Geometry check sheet. Reference: the model listing, model coordinates, mm. Face numbers are marked on the shaded views. A direction names the side the tool comes from. Round coordinates to 2 decimals unless told otherwise and drop trailing zeros. Write each loop counter-clockwise with the first axis right and the second up, starting at its lowest first coordinate (ties: lowest second). Pieces come first, ordered by that corner, then holes. Notation, with made-up numbers: (11.25, 0) -> (41.25, 0) arc R12 ccw to (41.25, 5) -> close; hole circle Ø6 at (43, 31.25). An arc over 180 degrees is marked (long way). Use a Markdown table: item, result.
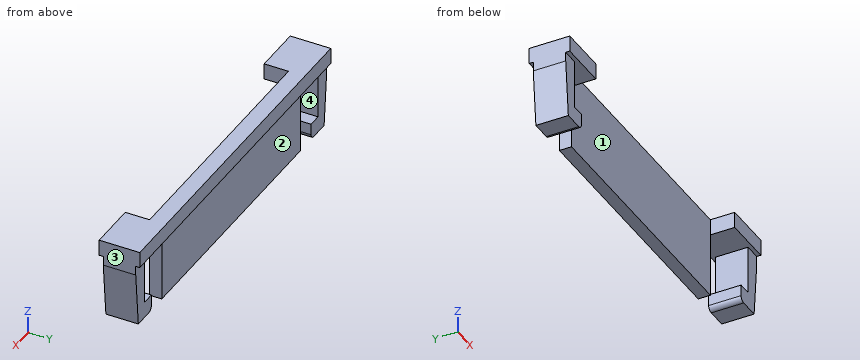
```python
from build123d import *

# Parameters (mm, degrees)
SKETCH1_W             = 22
SKETCH1_H             = 2.5
BOSS_EXTRUDE1_DEPTH   = 5
SKETCH2_W             = 22
SKETCH2_H             = 0.25
CUT_EXTRUDE1_DEPTH    = 4
SKETCH3_W             = 2
SKETCH3_H             = 2
CUT_EXTRUDE2_DEPTH    = 4
SKETCH5_W             = 16
SKETCH5_H             = 1.5
CUT_EXTRUDE3_DEPTH    = 5
SKETCH6_W             = 1.8
SKETCH6_H             = 1
BOSS_EXTRUDE2_DEPTH   = 2
FILLET1_R             = 0.3
CHAMFER1_SIZE2        = 0.3
CHAMFER1_SIZE         = 3.429015691
CHAMFER1_EDGE_2_SIZE2 = 0.3
CHAMFER1_EDGE_2_SIZE  = 3.429015691


with BuildPart() as part:
    # Sketch1 → Boss-Extrude1 (new body)
    with BuildSketch(Plane.XY):
        Rectangle(SKETCH1_W, SKETCH1_H)
    extrude(amount=BOSS_EXTRUDE1_DEPTH)

    # Sketch2 → Cut-Extrude1 (cut)
    with BuildSketch(Plane(origin=(0, 0, 0), x_dir=(-1, 0, 0), z_dir=(0, 0, -1))):
        with Locations((0, 1.125)):
            Rectangle(SKETCH2_W, SKETCH2_H)
        with Locations((0, -1.125)):
            Rectangle(SKETCH2_W, SKETCH2_H)
    extrude(amount=-CUT_EXTRUDE1_DEPTH, mode=Mode.SUBTRACT)

    # Sketch3 → Cut-Extrude2 (cut)
    with BuildSketch(Plane(origin=(0, 0, 0), x_dir=(-1, 0, 0), z_dir=(0, 0, -1))):
        with Locations((-9, 0)):
            Rectangle(SKETCH3_W, SKETCH3_H)
        with Locations((9, 0)):
            Rectangle(SKETCH3_W, SKETCH3_H)
    extrude(amount=-CUT_EXTRUDE2_DEPTH, mode=Mode.SUBTRACT)

    # Sketch5 → Cut-Extrude3 (cut)
    with BuildSketch(Plane(origin=(0, 0, 0), x_dir=(-1, 0, 0), z_dir=(0, 0, -1))):
        with Locations((0, -0.5)):
            Rectangle(SKETCH5_W, SKETCH5_H)
    extrude(amount=-CUT_EXTRUDE3_DEPTH, mode=Mode.SUBTRACT)

    # Sketch6 → Boss-Extrude2 (add)
    with BuildSketch(Plane(origin=(0, 1, 0), x_dir=(1, 0, 0), z_dir=(0, 1, 0))):
        with Locations((-10.1, -0.5)):
            Rectangle(SKETCH6_W, SKETCH6_H)
        with Locations((10.1, -0.5)):
            Rectangle(SKETCH6_W, SKETCH6_H)
    extrude(amount=-BOSS_EXTRUDE2_DEPTH)

    # Fillet1
    fillet1_edges = [part.edges().sort_by_distance(p)[0] for p in [
        (-9.2, 0, 0),
        (9.2, 0, 0),
    ]]
    fillet(fillet1_edges, radius=FILLET1_R)

    # Chamfer1
    chamfer1_edges = [part.edges().sort_by_distance(p)[0] for p in [
        (11, 0, 0),
    ]]
    chamfer(chamfer1_edges, length=CHAMFER1_SIZE, length2=CHAMFER1_SIZE2)

    # Chamfer1 edge 2
    chamfer1_edge_2_edges = [part.edges().sort_by_distance(p)[0] for p in [
        (-11, 0, 0),
    ]]
    chamfer(chamfer1_edge_2_edges, length=CHAMFER1_EDGE_2_SIZE, length2=CHAMFER1_EDGE_2_SIZE2)


solid = part.part
```
(1) Section check D-D on x = 2.75. Record the cut outline in (y, z), plus the area to 3 significant figures.
A:
| item | result |
|---|---|
| outline | (0.25, 0) -> (1, 0) -> (1, 4) -> (1.25, 4) -> (1.25, 5) -> (0.25, 5) -> close |
| area | 4.00 mm2 |
(2) Access from +Z, -Z, +X, -X, +Y, -Y to the whole of each face (thin tool, end or side, straight path). Record for the marked faces 1, 2, 3 and 4.
A:
| item | result |
|---|---|
| face 1 | +Z, -Z, -Y |
| face 2 | -Z, +X, -X, +Y |
| face 3 | +Z, -Z, +X, +Y, -Y |
| face 4 | +Y, -Y |
(3) Thickness scan on line 1 (X direction, y = 0.5, z = 0.55); line 2 (X direction, y = 0, z = 4.15); line 3 (X direction, y = 0.7, z = 1.15). Record the ranges inside material, lowest first.
A:
| item | result |
|---|---|
| line 1 | x = -10.75 to -9.2, -8 to 8, 9.2 to 10.75 |
| line 2 | x = -11 to -8, 8 to 11 |
| line 3 | x = -10.8 to -10, -8 to 8, 10 to 10.8 |
(4) Section check C-C on y = 0.75. Record the cut outline in (x, z), plus the area to 3 significant figures.
A:
| item | result |
|---|---|
| outline | (-11, 3.43) -> (-10.7, 0) -> (-9.5, 0) arc R0.3 ccw to (-9.2, 0.3) -> (-9.2, 1) -> (-10, 1) -> (-10, 4) -> (-8, 4) -> (-8, 0) -> (8, 0) -> (8, 4) -> (10, 4) -> (10, 1) -> (9.2, 1) -> (9.2, 0.3) arc R0.3 ccw to (9.5, 0) -> (10.7, 0) -> (11, 3.43) -> (11, 5) -> (-11, 5) -> close |
| area | 94.5 mm2 |
(5) Section check B-B on z = 2.55. Record the cut outline in (x, y).
A:
| item | result |
|---|---|
| outline | (-10.92, -1) -> (-10, -1) -> (-10, 1) -> (-10.92, 1) -> close; (-8, 0.25) -> (8, 0.25) -> (8, 1) -> (-8, 1) -> close; (10, -1) -> (10.92, -1) -> (10.92, 1) -> (10, 1) -> close |
(6) Gauge pin test, flat ends, axial feed: pin 1 Ø2 at (x, z) = (0, 1.5) entering from +Y; pin 2 Ø0.6 at (y, z) = (-0.5, 0.5) entering from -X; pin 3 Ø0.9 at (x, z) = (-10, 2.5) entering from -Y. Record the tip position at first contact, or that the pin passes through.
A:
| item | result |
|---|---|
| pin 1 | stops at y = 1 |
| pin 2 | stops at x = -10.77 |
| pin 3 | stops at y = -1 |
(7) Section check A-A on y = -0.8. Record the cut outline in (x, z).
A:
| item | result |
|---|---|
| outline | (-11, 3.43) -> (-10.7, 0) -> (-9.5, 0) arc R0.3 ccw to (-9.2, 0.3) -> (-9.2, 1) -> (-10, 1) -> (-10, 4) -> (-8, 4) -> (-8, 5) -> (-11, 5) -> close; (8, 4) -> (10, 4) -> (10, 1) -> (9.2, 1) -> (9.2, 0.3) arc R0.3 ccw to (9.5, 0) -> (10.7, 0) -> (11, 3.43) -> (11, 5) -> (8, 5) -> close |
